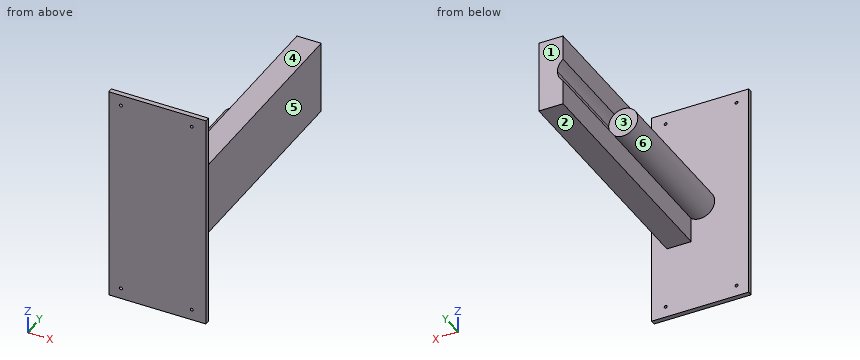
```python
from build123d import *

# Parameters (mm, degrees)
SKETCH1_W           = 200
SKETCH1_H           = 450
SKETCH1_R           = 3
BOSS_EXTRUDE1_DEPTH = 10
SKETCH2_R           = 30
BOSS_EXTRUDE2_DEPTH = 300
BOSS_EXTRUDE3_DEPTH = 500


with BuildPart() as part:
    # Sketch1 → Boss-Extrude1 (new body)
    with BuildSketch(Plane(origin=(0, 0, 0), x_dir=(1, 0, 0), z_dir=(0, 1, 0))):
        Rectangle(SKETCH1_W, SKETCH1_H)
        with Locations(Location((-75, 202.5, 0), (0, 0, 270))):
            Circle(SKETCH1_R, mode=Mode.SUBTRACT)
        with Locations(Location((71, 202.5, 0), (0, 0, 270))):
            Circle(SKETCH1_R, mode=Mode.SUBTRACT)
        with Locations(Location((71, -202.5, 0), (0, 0, 90))):
            Circle(SKETCH1_R, mode=Mode.SUBTRACT)
        with Locations(Location((-75, -202.5, 0), (0, 0, 90))):
            Circle(SKETCH1_R, mode=Mode.SUBTRACT)
    extrude(amount=BOSS_EXTRUDE1_DEPTH)

    # Sketch2 → Boss-Extrude2 (add)
    with BuildSketch(Plane(origin=(0, 10, 0), x_dir=(1, 0, 0), z_dir=(0, 1, 0))):
        with Locations(Location((0, 0, 0), (0, 0, 270))):
            Circle(SKETCH2_R)
    extrude(amount=BOSS_EXTRUDE2_DEPTH)

    # Sketch2_3 → Boss-Extrude3 (add)
    with BuildSketch(Plane(origin=(0, 10, 0), x_dir=(1, 0, 0), z_dir=(0, 1, 0))):
        with BuildLine():
            Line((18.394275911, 75), (18.394275911, 23.699169051))
            ThreePointArc((18.394275911, 23.699169051), (26.942793817, 13.194160122), (30, 0))
            ThreePointArc((30, 0), (26.942793817, -13.194160122), (18.394275911, -23.699169051))
            Line((18.394275911, -23.699169051), (18.394275911, -75))
            Line((18.394275911, -75), (68.394275911, -75))
            Line((68.394275911, -75), (68.394275911, 75))
            Line((68.394275911, 75), (18.394275911, 75))
        make_face()
    extrude(amount=BOSS_EXTRUDE3_DEPTH)


solid = part.part
```
The listing builds one solid part. Answer for the finished solid, in the listing's coordinates (mm). Face numbers are marked on the shaded views. A direction names the side the tool comes from. Coordinates: 2 decimals unless noted, no trailing zeros. Write each loop counter-clockwise with the first axis right and the second up, starting at its lowest first coordinate (ties: lowest second). Pieces come first, ordered by that corner, then holes. Notation, with made-up numbers: (50, 49) - (103, 49) arc R25 cw to (103, 74) - close; hole circle Ø1 at (10.25, 29.5). An arc over 180 degrees is marked (long way). Return JSON: item names as keys, results as strings. Group by question number.
1. Straight lines are drawn through the part: L1, parallel to X at y = 5.5, z = -202.5; L2, parallel to Y at x = -54.5, z = 131.5; L3, parallel to X at y = 67, z = 65. For each, find the intervals that lie inside material, in ascending order.
2. Determine the mould class of the marked faces 4, 5 and 6 for opening direction X: released by +X, released by -X, zero draft, split by the parting line, or undercut.
3. A cutting plane is placed at D-D, the plane y = 61. Determine the outline of the cut face in (x, z), plus the area to 3 significant figures.
4. Given pin 1 (1.5 mm diameter, centred on x = 15, y = 152, fed in from +Z); pin 2 (1.5 mm diameter, centred on x = -28.5, y = 286.5, fed in from -Z); pin 3 (3 mm diameter, centred on x = 9, z = -96, fed in from -Y); pin 4 (6 mm diameter, centred on y = 345.5, z = 61.5, fed in from -X), each flat-ended and moving along its own axis, determine where each tip first touches the part or whether it passes through.
5. A cutting plane is placed at A-A, the plane z = -38.5. Determine the outline of the cut face in (x, y), plus the area to 3 significant figures.
6. A cutting plane is placed at B-B, the plane y = 445.5. Determine the outline of the cut face in (x, z), plus the area to 3 significant figures.
7. A cutting plane is placed at C-C, the plane x = 6. Determine the outline of the cut face in (y, z).
8. Which of the six approach directions +Z, -Z, +X, -X, +Y, -Y give full straight-line access (tool end or side, diameter ignored) to the marked faces 1, 2 and 3?
Ans:
{
 "1": {"L1": "-100 to -78, -72 to 68, 74 to 100", "L2": "0 to 10", "L3": "18.39 to 68.39"},
 "2": {"face 4": "zero draft", "face 5": "released by +X", "face 6": "undercut"},
 "3": {"outline": "(18.39, -75) - (68.39, -75) - (68.39, 75) - (18.39, 75) - (18.39, 23.7) arc R30 ccw (long way) to (18.39, -23.7) - close", "area": "9,940 mm²"},
 "4": {"pin 1": "z = 26.4", "pin 2": "z = -11.4", "pin 3": "y = 0", "pin 4": "x = 18.39"},
 "5": {"outline": "(-100, 0) - (100, 0) - (100, 10) - (68.39, 10) - (68.39, 510) - (18.39, 510) - (18.39, 10) - (-100, 10) - close", "area": "27,000 mm²"},
 "6": {"outline": "(18.39, -75) - (68.39, -75) - (68.39, 75) - (18.39, 75) - (18.39, 23.7) arc R30 cw to (18.39, -23.7) - close", "area": "7,120 mm²"},
 "7": {"outline": "(0, -225) - (10, -225) - (10, -29.39) - (310, -29.39) - (310, 29.39) - (10, 29.39) - (10, 225) - (0, 225) - close"},
 "8": {"face 1": "+Z, -Z, +X, -X, +Y", "face 2": "-Z, +X, -X, +Y", "face 3": "-X, +Y"}
}
